Autodesk Fusion 360 part; units mm, degrees
sketch "Sketch1" plane through (0, 0, 0) normal (0, 1, 0) x (1, 0, 0)
  line L0 (-18.5178, -25) -> (-4.0178, -25)
  line L1 (-4.0178, -25) -> (-4.0178, 5)
  line L2 (-4.0178, 5) -> (-18.5178, 5)
  line L3 (-18.5178, 5) -> (-18.5178, -25)
  line L4 (-16.5178, 5) -> (-6.0178, 5)
  line L5 (-6.0178, 5) -> (-6.0178, -24)
  line L6 (-6.0178, -24) -> (-16.5178, -24)
  line L7 (-16.5178, -24) -> (-16.5178, 5)
  dimension "d1" = 14.5
  dimension "d2" = 30
  dimension "d3" = 10.5
  dimension "d4" = 2
  dimension "d5" = 1
extrude "Extrude1" add sketch "Sketch1" along normal blind 60 contours L0 L1 L2 L3 L5 L6 L7
fillet "Fillet1" radius 5 1 edges at (-5.0178, 0, -5)
fillet "Fillet2" radius 5 1 edges at (-17.5178, 0, -5)
fillet "Fillet3" radius 5 1 edges at (-17.5178, 60, -5)
fillet "Fillet4" radius 5 1 edges at (-5.0178, 60, -5)
Could you check a few things on this model? Use its own coordinates, in mm. A direction names the side the tool comes from. Give positions to 0.01 mm unless a question says otherwise; leave off trailing zeros. Order: outer loops, then holes, each group sorted by start corner. A loop starts at its lowest first (then second) coordinate and runs counter-clockwise, first axis right, second up. Notation, with made-up numbers: (-16, -27.5) - (23, -27.5) arc R30 cw to (23, 0.5) - close; hole circle Ø2 at (3, 39.5). An arc over 180 degrees is marked (long way). Return JSON: item names as keys, results as strings. Group by question number.
Q1. Suppose I cut it at A-A, the plane z = 14.25. Please give me the cut outline in (x, y).
Q2. Please list where these lines run through material, in increasing order: line 1 along X through (y, z) = (8.5, 8.25); line 2 along Z through (x, y) = (-15, 44). Write a range as [from, to].
Q3. Will this pin go through, and if not, where does the flat tip stop? pin 1 Ø3 at (x, y) = (-11, 33) entering from -Z.
Q4. Suppose I cut it at B-B, the plane y = 30.5. Please give me the cut outline in (x, z).
Q5. Which directions (+Z, -Z, +X, -X, +Y, -Y) give clear straight access to the entire face, cutting with the end or side of a thin tool? Please do faces 1 (the face through (-4.018, 30, 10)), 2 (the face through (-11, 30, 24)).
Q6. Suppose I cut it at C-C, the plane x = -9.25. Please give me the cut outline in (y, z), and give its area (3 significant figures).
Q7. Thinking about a two-plate mould opening in X: for faces 3 (the face through (-16.518, 30, 10)), 4 (the face through (-6.018, 30, 9)), 5 (the face through (-5, 59, -3)), 6 (the face through (-18.518, 30, 10)), which applies, pulls with the +X half, pulls with the -X half, needs draft (parallel to the pull), parting line crosses it, or undercut?
Resolved:
{
 "1": {"outline": "(-18.52, 0) - (-16.52, 0) - (-16.52, 60) - (-18.52, 60) - close; (-6.02, 0) - (-4.02, 0) - (-4.02, 60) - (-6.02, 60) - close"},
 "2": {"line 1": "x = [-18.52, -16.52], [-6.02, -4.02]", "line 2": "z = [24, 25]"},
 "3": {"pin 1": "stops at z = 24"},
 "4": {"outline": "(-18.52, -5) - (-16.52, -5) - (-16.52, 24) - (-6.02, 24) - (-6.02, -5) - (-4.02, -5) - (-4.02, 25) - (-18.52, 25) - close"},
 "5": {"face 1": "+Z, -Z, +X, +Y, -Y", "face 2": "-Z, +Y, -Y"},
 "6": {"outline": "(0, 24) - (60, 24) - (60, 25) - (0, 25) - close", "area": "60.0 mm2"},
 "7": {"face 3": "undercut", "face 4": "undercut", "face 5": "needs draft", "face 6": "pulls with the -X half"}
}
